The drawing under review shows one solid part. Ordinate dimensions are in mm from its lowest x, y, z. A direction names the side the tool comes from. Coordinates: 2 decimals unless noted, no trailing zeros. Write each loop counter-clockwise with the first axis right and the second up, starting at its lowest first coordinate (ties: lowest second). Pieces come first, ordered by that corner, then holes. Notation, with made-up numbers: (-24, 6.5) - (-19, 6.5) arc R5 cw to (-19, 12.5) - close; hole circle Ø5 at (-27.5, -14). An arc over 180 degrees is marked (long way). Put each result on its own line as item: value. Start each with the question number.
Item 1: Consider section D-D on y = 57.5. Give the boundary of the cut face in (x, z) (1 decimal).
Item 2: Consider section A-A on z = 12.75. Give the boundary of the cut face in (x, y) (1 decimal), then the cut area to 3 significant figures.
Item 3: Consider section C-C on z = 5. Give the boundary of the cut face in (x, y) (1 decimal).
Item 4: For pin 1 (12.5 mm diameter, centred on x = 30.5, z = 15, fed in from -Y); pin 2 (1.5 mm diameter, centred on x = 31.5, y = 64, fed in from -Z); pin 3 (3 mm diameter, centred on y = 11, z = 21, fed in from -X), all flat-tipped, find the tip position at first contact; note any pin that passes through.
Item 5: To check wall thickness, follow L1, parallel to Y at x = 10.5, z = 11; L2, parallel to X at y = 54.5, z = 20.75 (1 decimal); L3, parallel to X at y = 66, z = 15.25 (1 decimal). State the ranges of each line that lie inside material, in increasing order. Write a range as [from, to].
Item 6: Mouldability with a two-part tool opening along X and no side actions: class the marked faces 3, 4, 5 and 6 as pulls with the +X half, pulls with the -X half, needs draft (parallel to the pull), parting line crosses it, or undercut.
Item 7: Machinability: for the marked faces 1 and 2, which of the approach directions +Z, -Z, +X, -X, +Y, -Y give a long, thin tool a straight path to every point of the face, cutting with its end or side? Answer none if there is none.
Item 8: Consider section B-B on y = 31.5. Give the boundary of the cut face in (x, z) (1 decimal), then the cut area to 3 significant figures.
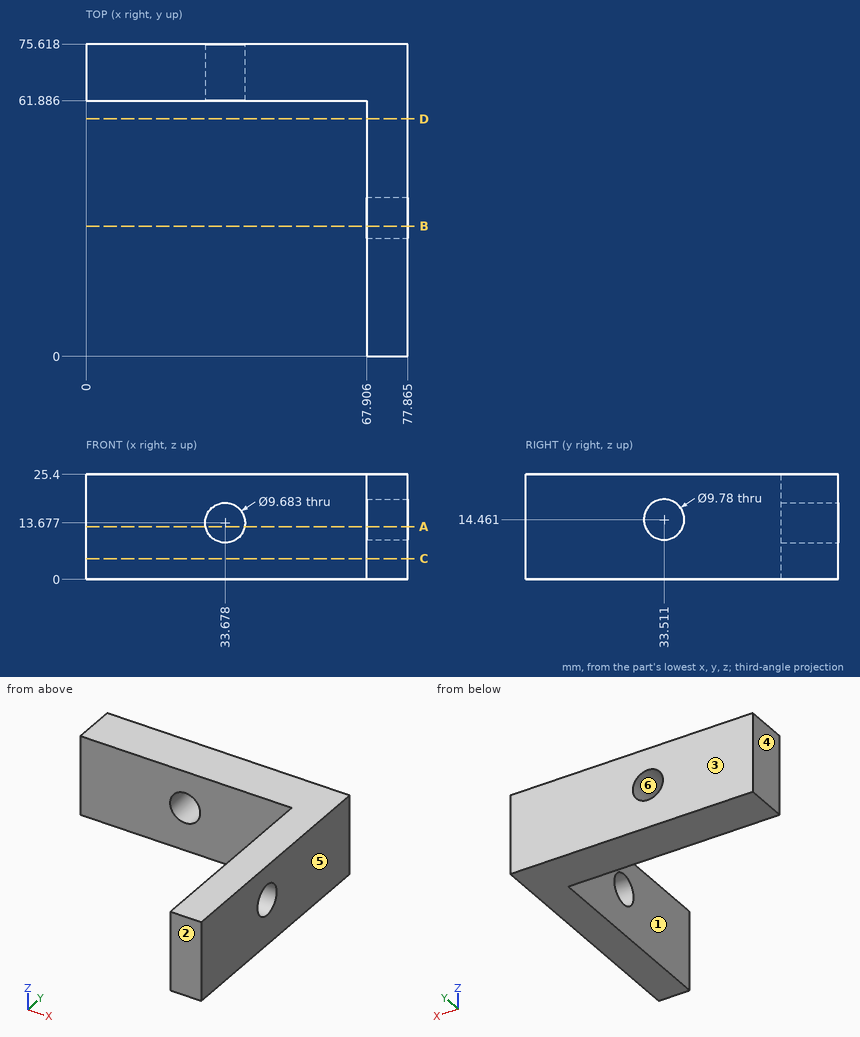
Report:
1. outline: (67.9, 0) - (77.9, 0) - (77.9, 25.4) - (67.9, 25.4) - close
2. outline: (0, 61.9) - (28.9, 61.9) - (28.9, 75.6) - (0, 75.6) - close; (38.4, 61.9) - (67.9, 61.9) - (67.9, 38.1) - (77.9, 38.1) - (77.9, 75.6) - (38.4, 75.6) - close; (67.9, 0) - (77.9, 0) - (77.9, 28.9) - (67.9, 28.9) - close
2. area: 1,460 mm²
3. outline: (0, 61.9) - (67.9, 61.9) - (67.9, 0) - (77.9, 0) - (77.9, 75.6) - (0, 75.6) - close
4. pin 1: y = 61.89
4. pin 2: z = 0
4. pin 3: x = 67.91
5. L1: [61.89, 75.62]
5. L2: [67.9, 77.9]
5. L3: [0, 29.1], [38.3, 77.9]
6. face 3: needs draft
6. face 4: pulls with the -X half
6. face 5: pulls with the +X half
6. face 6: undercut
7. face 1: +Z, -Z, -X, -Y
7. face 2: +Z, -Z, +X, -X, -Y
8. outline: (67.9, 0) - (77.9, 0) - (77.9, 10) - (67.9, 10) - close; (67.9, 18.9) - (77.9, 18.9) - (77.9, 25.4) - (67.9, 25.4) - close
8. area: 164 mm²
